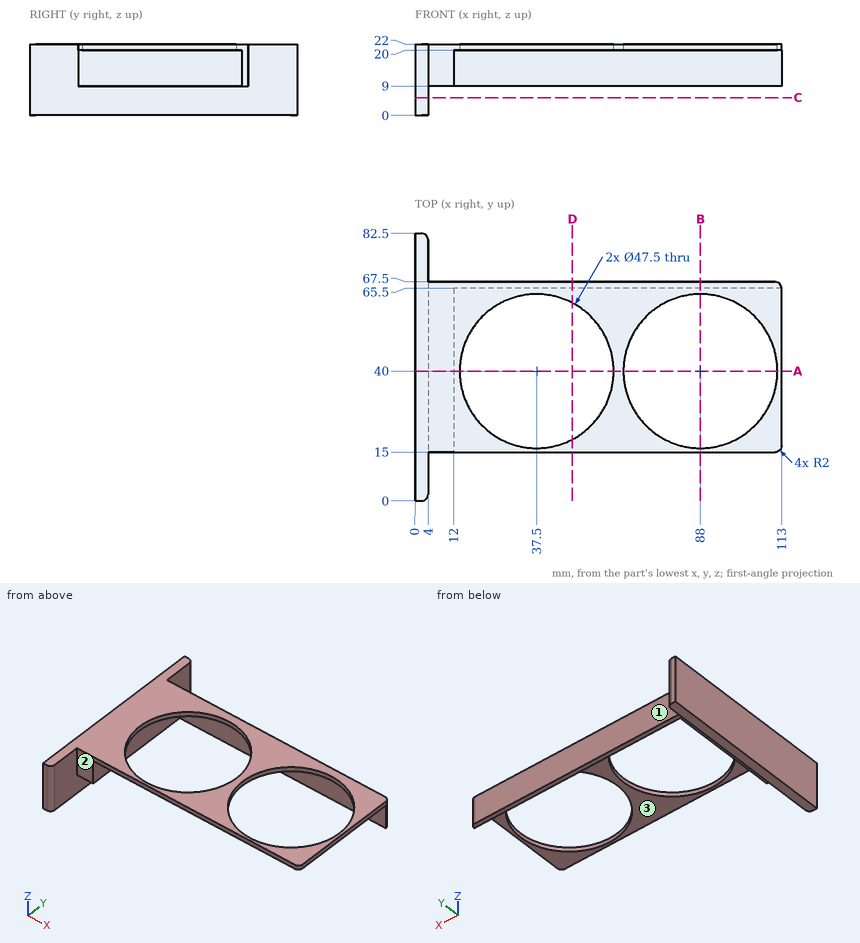
Study the drawing (mm; zero at the part's minimum x, y, z) and answer. A direction names the side the tool comes from. Coordinates: 2 decimals unless noted, no trailing zeros. Write each loop counter-clockwise with the first axis right and the second up, starting at its lowest first coordinate (ties: lowest second). Pieces come first, ordered by that corner, then holes. Notation, with made-up numbers: (42, -39) - (93, -39) arc R11 cw to (93, -27) - close; hole circle Ø6 at (52, 78). An arc over 180 degrees is marked (long way). Return JSON: item names as keys, results as strings. Group by question number.
1. A cutting plane is placed at C-C, the plane z = 5.5. Determine the outline of the cut face in (x, y).
2. A cutting plane is placed at D-D, the plane x = 48.5. Determine the outline of the cut face in (y, z).
3. Straight lines are drawn through the part: L1, parallel to Y at x = 37.5, z = 20.4; L2, parallel to Z at x = 75, y = 60; L3, parallel to X at y = 9, z = 14. For each, find the intervals that lie inside material, in ascending order.
4. A cutting plane is placed at B-B, the plane x = 88. Determine the outline of the cut face in (y, z), plus the area to 3 significant figures.
5. Which of the six approach directions +Z, -Z, +X, -X, +Y, -Y give full straight-line access (tool end or side, diameter ignored) to the marked faces 1, 2 and 3?
6. A cutting plane is placed at A-A, the plane y = 40. Determine the outline of the cut face in (x, z), plus the area to 3 significant figures.
7. Given pin 1 (1 mm diameter, centred on x = 27, z = 17, fed in from -Y); pin 2 (6.5 mm diameter, centred on x = 55, z = 18, fed in from +Y), each flat-ended and moving along its own axis, determine where each tip first touches the part or whether it passes through.
Ans:
{
 "1": {"outline": "(0, 0) - (2, 0) arc R2 ccw to (4, 2) - (4, 80.5) arc R2 ccw to (2, 82.5) - (0, 82.5) - close"},
 "2": {"outline": "(15, 20) - (18.95, 20) - (18.95, 22) - (15, 22) - close; (61.05, 20) - (65.5, 20) - (65.5, 9) - (67.5, 9) - (67.5, 22) - (61.05, 22) - close"},
 "3": {"L1": "15 to 16.25, 63.75 to 67.5", "L2": "20 to 22", "L3": "0 to 4"},
 "4": {"outline": "(15, 20) - (16.25, 20) - (16.25, 22) - (15, 22) - close; (63.75, 20) - (65.5, 20) - (65.5, 9) - (67.5, 9) - (67.5, 22) - (63.75, 22) - close", "area": "32.0 mm²"},
 "5": {"face 1": "+Z, -Z, +X, +Y", "face 2": "+Z, -Z, +X, -Y", "face 3": "-Z, +X, -Y"},
 "6": {"outline": "(0, 0) - (4, 0) - (4, 9) - (12, 9) - (12, 20) - (13.75, 20) - (13.75, 22) - (0, 22) - close; (61.25, 20) - (64.25, 20) - (64.25, 22) - (61.25, 22) - close; (111.75, 20) - (113, 20) - (113, 22) - (111.75, 22) - close", "area": "204 mm²"},
 "7": {"pin 1": "y = 65.5", "pin 2": "y = 67.5"}
}
